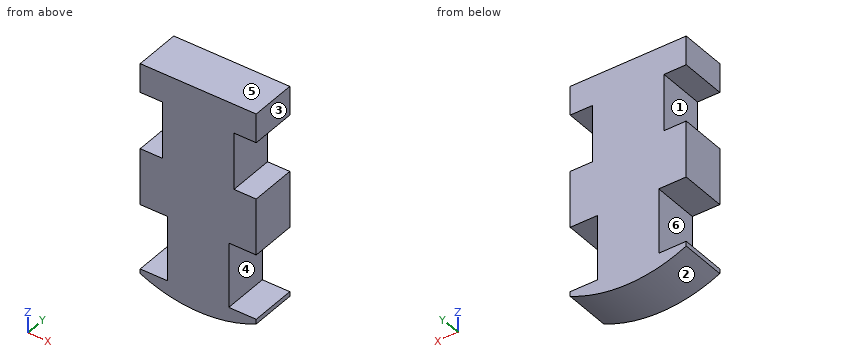
from build123d import *

# Parameters (mm, degrees)
BOSS_EXTRUDE1_DEPTH = 60.706


with BuildPart() as part:
    # Sketch2 → Boss-Extrude1 (new body)
    with BuildSketch(Plane(origin=(0, 0, 0), x_dir=(1, 0, 0), z_dir=(0, 1, 0))):
        with BuildLine():
            Line((-76.2, -147.828), (76.2, -147.828))
            Line((76.2, -147.828), (76.2, -109.728))
            Line((76.2, -109.728), (46.99, -109.728))
            Line((46.99, -109.728), (46.99, -35.052))
            Line((46.99, -35.052), (76.2, -35.052))
            Line((76.2, -35.052), (76.2, 39.116))
            Line((76.2, 39.116), (40.132, 39.116))
            Line((40.132, 39.116), (40.132, 124.46))
            Line((40.132, 124.46), (76.2, 124.46))
            Line((76.2, 124.46), (76.2, 130.671705137))
            ThreePointArc((76.2, 130.671705137), (0, 147.828), (-76.2, 130.671705137))
            Line((-76.2, 130.671705137), (-76.2, 124.46))
            Line((-76.2, 124.46), (-40.132, 124.46))
            Line((-40.132, 124.46), (-40.132, 39.116))
            Line((-40.132, 39.116), (-76.2, 39.116))
            Line((-76.2, 39.116), (-76.2, -35.052))
            Line((-76.2, -35.052), (-46.99, -35.052))
            Line((-46.99, -35.052), (-46.99, -109.728))
            Line((-46.99, -109.728), (-76.2, -109.728))
            Line((-76.2, -109.728), (-76.2, -147.828))
        make_face()
    extrude(amount=BOSS_EXTRUDE1_DEPTH)


solid = part.part
Work out the finished part from the listing and answer in its coordinate system (mm). Face numbers are marked on the shaded views. A direction names the side the tool comes from. Give positions to 0.01 mm unless a question says otherwise; leave off trailing zeros. Loops run counter-clockwise (first coordinate to the right, second up) from the corner with the lowest first, then second, coordinate; pieces in that order, holes last. Notation, with made-up numbers: (0, -2.5) - (39, -2.5) arc R16 cw to (39, 19.5) - close; hole circle Ø6 at (47, 78.5). An arc over 180 degrees is marked (long way). Answer in a Markdown table with one row per item.
(1) Consider L1, parallel to Z at x = 56.5, y = 8; L2, parallel to Z at x = -48, y = 20.5; L3, parallel to X at y = 37, z = 83. Determine where each line is inside the solid, lowest interval first. Write a range as [from, to].
Results list:
| item | result |
|---|---|
| L1 | z = [-138.61, -124.46], [-39.12, 35.05], [109.73, 147.83] |
| L2 | z = [-141.23, -124.46], [-39.12, 35.05], [109.73, 147.83] |
| L3 | x = [-46.99, 46.99] |
(2) Section A-A (y = 12) is taken. Give the vertices of the cut face in (x, z), and give its area (3 significant figures).
Results list:
| item | result |
|---|---|
| outline | (-76.2, -130.67) arc R177.8 ccw to (76.2, -130.67) - (76.2, -124.46) - (40.13, -124.46) - (40.13, -39.12) - (76.2, -39.12) - (76.2, 35.05) - (46.99, 35.05) - (46.99, 109.73) - (76.2, 109.73) - (76.2, 147.83) - (-76.2, 147.83) - (-76.2, 109.73) - (-46.99, 109.73) - (-46.99, 35.05) - (-76.2, 35.05) - (-76.2, -39.12) - (-40.13, -39.12) - (-40.13, -124.46) - (-76.2, -124.46) - close |
| area | 33,700 mm² |
(3) Section B-B (z = 50) is taken. Give the vertices of the cut face in (x, y).
Results list:
| item | result |
|---|---|
| outline | (-46.99, 0) - (46.99, 0) - (46.99, 60.71) - (-46.99, 60.71) - close |
(4) For a pull along Z with two mould halves and no side action, classify the marked faces 1, 2 and 3 as pulls with the +Z half, pulls with the -Z half, needs draft (parallel to the pull), parting line crosses it, or undercut.
Results list:
| item | result |
|---|---|
| face 1 | undercut |
| face 2 | pulls with the -Z half |
| face 3 | needs draft |
(5) A tool of negligible diameter and unlimited length cuts with its end or side. For the marked faces 4, 5 and 6, from which of +Z, -Z, +X, -X, +Y, -Y can it reach the whole face along a straight path? Write none if from no direction.
Results list:
| item | result |
|---|---|
| face 4 | +X, +Y, -Y |
| face 5 | +Z, +X, -X, +Y, -Y |
| face 6 | -X, +Y, -Y |
(6) Flat-ended cylindrical pins translate along their axes: pin 1 Ø6 at (x, z) = (33.5, 47) entering from -Y; pin 2 Ø3 at (y, z) = (27.5, -97) entering from +X; pin 3 Ø18 at (y, z) = (34.5, -99) entering from -X; pin 4 Ø23.5 at (x, y) = (58, 29) entering from -Z. Find the tip coordinate at first contact, or state that the pin passes through.
Results list:
| item | result |
|---|---|
| pin 1 | stops at y = 0 |
| pin 2 | stops at x = 40.13 |
| pin 3 | stops at x = -40.13 |
| pin 4 | stops at z = -141.71 |
